```python
from build123d import *

# Parameters (mm, degrees)
SKETCH1_W           = 49.9618
SKETCH1_H           = 69.0118
BOSS_EXTRUDE1_DEPTH = 1.1566
SKETCH3_W           = 43.199747393
SKETCH3_H           = 57.599795215
CUT_EXTRUDE1_DEPTH  = 0.1


with BuildPart() as part:
    # Sketch1 → Boss-Extrude1 (new body)
    with BuildSketch(Plane.XY.offset(8.79254995)):
        with Locations((2.257083431, -61.428094771)):
            Rectangle(SKETCH1_W, SKETCH1_H)
    extrude(amount=BOSS_EXTRUDE1_DEPTH)

    # Sketch3 → Cut-Extrude1 (cut)
    with BuildSketch(Plane.XY.offset(9.94914995)):
        with Locations((2.256996925, -64.104049821)):
            Rectangle(SKETCH3_W, SKETCH3_H)
    extrude(amount=-CUT_EXTRUDE1_DEPTH, mode=Mode.SUBTRACT)


solid = part.part
```
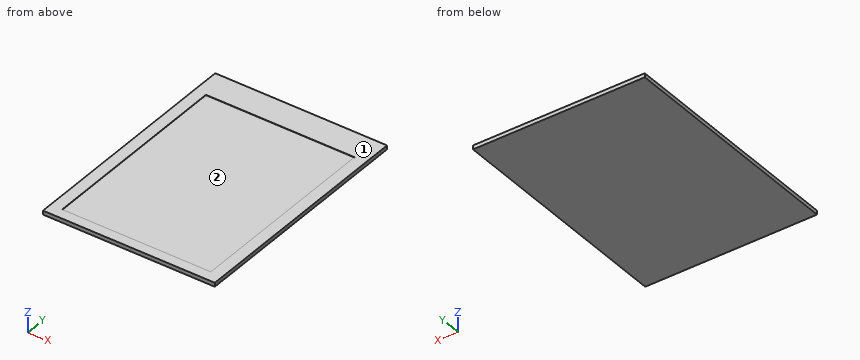
Here's how the part is built. I have some questions about the finished solid (model axes, mm). Face numbers are marked on the shaded views. Coordinates: 2 decimals unless noted, no trailing zeros. Order: outer loops, then holes, each group sorted by start corner. A loop starts at its lowest first (then second) coordinate and runs counter-clockwise, first axis right, second up. Notation, with made-up numbers: (15.5, 41.5) -> (47.5, 41.5) arc R23 cw to (47.5, 78.5) -> close; hole circle Ø5 at (-22.5, 0). An arc over 180 degrees is marked (long way). Return JSON: item names as keys, results as strings.
1) If I drill on probe 1 along Z at (x, y) = (-7, -57); probe 2 along X at (y, z) = (-47, 9.9), over which ranges is the centre line in solid material (lowest first)?
Conclusion:
{"probe 1": "z = 8.79 to 9.85", "probe 2": "x = -22.72 to -19.34, 23.86 to 27.24"}
2) I'm going to push a flat-ended pin straight in: P1, Ø2, axis at x = -14.5, y = -56.5, coming from the +Z side. Where does the tip first touch, or does it pass through?
Conclusion:
{"P1": "stops at z = 9.85"}
3) If we section it at A-A on y = -54: List the corners of the cut face in (x, z) for me.
Conclusion:
{"outline": "(-22.72, 8.79) -> (27.24, 8.79) -> (27.24, 9.95) -> (23.86, 9.95) -> (23.86, 9.85) -> (-19.34, 9.85) -> (-19.34, 9.95) -> (-22.72, 9.95) -> close"}
4) If we section it at B-B on x = 7: List the corners of the cut face in (y, z) for me.
Conclusion:
{"outline": "(-95.93, 8.79) -> (-26.92, 8.79) -> (-26.92, 9.95) -> (-35.3, 9.95) -> (-35.3, 9.85) -> (-92.9, 9.85) -> (-92.9, 9.95) -> (-95.93, 9.95) -> close"}
5) Thinking about a two-plate mould opening in Y: for the marked faces 1 and 2, which applies, +Y half, -Y half, draft (parallel to the pull), parting line (faces both ways), or undercut?
Conclusion:
{"face 1": "draft", "face 2": "undercut"}
